Read the model definition and answer for the solid it produces. Units are mm, in the model's axes. A direction names the side the tool comes from. Coordinates: 2 decimals unless noted, no trailing zeros. Write each loop counter-clockwise with the first axis right and the second up, starting at its lowest first coordinate (ties: lowest second). Pieces come first, ordered by that corner, then holes.
1) The part is cut by section B-B (z = 20). Determine the outline of the cut face in (x, y), then the cut area to 3 significant figures.
2) Find the intervals of material crossed by line 1 (Y direction, x = 72.5, z = 20.5); line 2 (X direction, y = -58, z = 7.5); line 3 (X direction, y = -92, z = 3.5), in increasing order.
3) The part is cut by section C-C (x = 11). Determine the outline of the cut face in (y, z).
4) Determine the mould class of faces 1 (the face through (58.8, -108.7, 28.9)), 2 (the face through (58.909, -122.756, 1.915)), 3 (the face through (-90.853, -78, 9)) for opening direction X: +X half, -X half, draft (parallel to the pull), parting line (faces both ways), or undercut.
5) Which of the six approach directions +Z, -Z, +X, -X, +Y, -Y give full straight-line access (tool end or side, diameter ignored) to faces 4 (the face through (-79, -78, 12.785)), 5 (the face through (-55.43, -113.26, 28.55)), 6 (the face through (59.036, -122.756, 7.391))?
6) Each of these flat-tipped pins is pushed along its axis until it touches: pin 1 Ø7.5 at (x, y) = (87, -95) entering from +Z; pin 2 Ø4 at (x, y) = (8, -121) entering from -Z; pin 3 Ø10 at (x, y) = (-85, -98.5) entering from -Z. Where does it stop, or does it pass through?
7) The part is cut by section A-A (y = -53). Determine the outline of the cut face in (x, z), then the cut area to 3 significant figures.
from build123d import *

# Parameters (mm, degrees)
PAD005_DEPTH    = 80
PAD006_DEPTH    = 8
PAD007_DEPTH    = 80
SKETCH011_R     = 6.937769
PAD008_DEPTH    = 1
SKETCH012_R     = 4.849298
SKETCH012_R_2   = 4.845408
PAD009_DEPTH    = 9
SKETCH013_R     = 1.431776
SKETCH013_R_2   = 1.476283
POCKET002_DEPTH = 5
PAD013_DEPTH    = 8


with BuildPart() as part:
    # Sketch008 → Pad005 (new body)
    with BuildSketch(Plane.XZ):
        Polygon((-81.828072, 16.941692), (-81.828072, 12.784613), (-75.591271, 12.784613), (-75.591271, 6.484819), (-81.863884, 6.484819), (-81.863884, 0.165597), (-90.85344, 0.165597), (-90.85344, 17.078894), align=None)
    extrude(amount=PAD005_DEPTH)

    # Sketch009 (on Face10 of Pad005) → Pad006 (join)
    with BuildSketch(Plane.XZ.offset(80)):
        with BuildLine():
            Line((-90.918877, 0), (-90.918877, 16.993577))
            Line((-90.918877, 16.993577), (-81.447352, 16.993577))
            ThreePointArc((-41.135882, 46.312654), (-74.731967, 50.132561), (-81.447352, 16.993577))
            Line((-41.135882, 46.312654), (0, 46.312654))
            Line((41.135882, 46.312654), (0, 46.312654))
            ThreePointArc((81.447352, 16.993577), (74.731967, 50.132561), (41.135882, 46.312654))
            Line((90.918877, 16.993577), (81.447352, 16.993577))
            Line((90.918877, 0), (90.918877, 16.993577))
            Line((68.692482, 0), (90.918877, 0))
            Line((44.563099, 25.81838), (68.692482, 0))
            Line((0, 25.81838), (44.563099, 25.81838))
            Line((0, 25.81838), (-44.563099, 25.81838))
            Line((-44.563099, 25.81838), (-68.692482, 0))
            Line((-68.692482, 0), (-90.918877, 0))
        make_face()
    extrude(amount=PAD006_DEPTH)

    # Sketch010 (on Face5 of Pad006) → Pad007 (join)
    with BuildSketch(Plane(origin=(0, -80, 0), x_dir=(1, 0, 0), z_dir=(0, 1, 0))):
        Polygon((81.838326, 0), (81.838326, -6.340793), (75.515793, -6.340793), (75.515793, -12.713724), (81.722115, -12.713724), (81.722115, -16.992775), (90.928337, -16.992775), (90.928337, 0), align=None)
    extrude(amount=PAD007_DEPTH)

    # Sketch011 (on Face5 of Pad007) → Pad008 (join)
    with BuildSketch(Plane(origin=(0, -80, 0), x_dir=(1, 0, 0), z_dir=(0, 1, 0))):
        with Locations((-59.983959, -30.058937)):
            Circle(SKETCH011_R)
        with Locations((59.983959, -30.058937)):
            Circle(SKETCH011_R)
    extrude(amount=PAD008_DEPTH)

    # Sketch012 (on Face39 of Pad008) → Pad009 (join)
    with BuildSketch(Plane(origin=(0, -79, 0), x_dir=(1, 0, 0), z_dir=(0, 1, 0))):
        with Locations((-60.056812, -30.004847)):
            Circle(SKETCH012_R)
        with Locations((59.971668, -30.024326)):
            Circle(SKETCH012_R_2)
    extrude(amount=PAD009_DEPTH)

    # Sketch013 (on Face43 of Pad009) → Pocket002 (cut)
    with BuildSketch(Plane(origin=(0, -70, 0), x_dir=(1, 0, 0), z_dir=(0, 1, 0))):
        with Locations((-60.000607, -29.970469)):
            Circle(SKETCH013_R)
        with Locations((60.014935, -30.002989)):
            Circle(SKETCH013_R_2)
    extrude(amount=-POCKET002_DEPTH, mode=Mode.SUBTRACT)

    # Sketch019 (on Face34 of Pocket002) → Pad013 (join)
    with BuildSketch(Plane.XZ.offset(88)):
        Polygon((-85.702133, 5.402917), (-85.702133, -2.272559), (-60.321888, -2.272559), (-57.456371, 6.221634), (-65.336533, 12.054996), align=None)
        Polygon((85.702133, 5.402917), (85.702133, -2.272559), (60.321888, -2.272559), (57.456371, 6.221634), (65.336533, 12.054996), align=None)
    extrude(amount=-PAD013_DEPTH)


with BuildPart() as part_1:
    # Body001 placement: moved
    add(part.part.moved(Location((0, -38.7, 0))))


solid = part_1.part
Reported:
1. outline: (-82.99, -126.7) - (-50, -126.7) - (-50, -118.7) - (-82.99, -118.7) - close; (50, -126.7) - (82.99, -126.7) - (82.99, -118.7) - (50, -118.7) - close
1. area: 528 mm2
2. line 1: y = -126.7 to -118.7
2. line 2: x = -90.85 to -75.59, 75.52 to 90.93
2. line 3: x = -90.85 to -81.86, 81.84 to 90.93
3. outline: (-126.7, 25.82) - (-118.7, 25.82) - (-118.7, 46.31) - (-126.7, 46.31) - close
4. face 1: draft
4. face 2: undercut
4. face 3: -X half
5. face 4: +Z, +Y
5. face 5: +Y
5. face 6: +Y, -Y
6. pin 1: stops at z = 16.99
6. pin 2: stops at z = 25.82
6. pin 3: stops at z = 0.17
7. outline: (-90.85, 0.17) - (-81.86, 0.17) - (-81.86, 6.48) - (-75.59, 6.48) - (-75.59, 12.78) - (-81.83, 12.78) - (-81.83, 16.94) - (-90.85, 17.08) - close; (75.52, 6.34) - (81.84, 6.34) - (81.84, 0) - (90.93, 0) - (90.93, 16.99) - (81.72, 16.99) - (81.72, 12.71) - (75.52, 12.71) - close
7. area: 386 mm2
